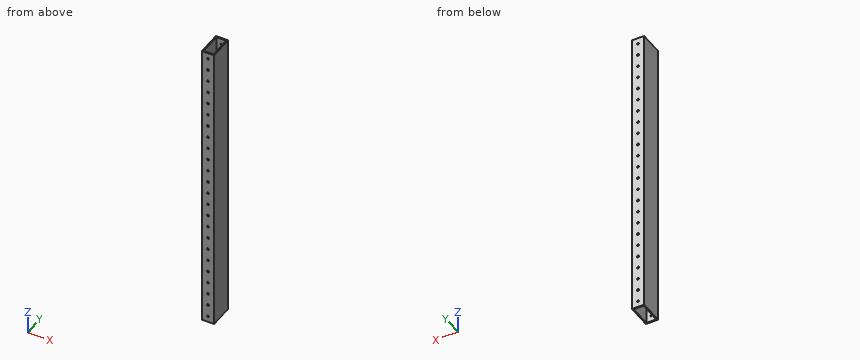
Autodesk Inventor part; units mm, degrees
ref_plane "YZ Plane" through (0, 0, 0) normal (1, 0, 0) x (0, 1, 0)
ref_plane "XZ Plane" through (0, 0, 0) normal (0, 1, 0) x (-1, 0, 0)
ref_plane "XY Plane" through (0, 0, 0) normal (0, 0, 1) x (1, 0, 0)
sketch "Sketch1" plane through (0, 0, 0) normal (0, 0, 1) x (1, 0, 0)
  line L0 (0, 0) -> (25.4, 0)
  line L1 (25.4, 0) -> (25.4, 50.8)
  line L2 (25.4, 50.8) -> (0, 50.8)
  line L3 (0, 50.8) -> (0, 0)
  line L4 (2.54, 2.54) -> (22.86, 2.54)
  line L5 (22.86, 2.54) -> (22.86, 48.26)
  line L6 (22.86, 48.26) -> (2.54, 48.26)
  line L7 (2.54, 48.26) -> (2.54, 2.54)
  dimension "d0" = 25.4
  dimension "d1" = 50.8
  dimension "d2" = 2.54
extrude "Extrusion1" add sketch "Sketch1" along normal blind 609.6
sketch "Sketch2" plane through (0, 50.8, 0) normal (0, 1, 0) x (1, 0, 0)
  line L0 (25.4, -609.6) -> (0, -609.6)
  line L1 (0, 0) -> (0, -609.6)
  point P0 (12.7, -596.9)
  point P1 (12.7, -571.5)
  point P2 (12.7, -546.1)
  point P3 (12.7, -520.7)
  point P4 (12.7, -495.3)
  point P5 (12.7, -469.9)
  point P6 (12.7, -444.5)
  point P7 (12.7, -419.1)
  point P8 (12.7, -393.7)
  point P9 (12.7, -368.3)
  point P10 (12.7, -342.9)
  point P11 (12.7, -317.5)
  point P12 (12.7, -292.1)
  point P13 (12.7, -266.7)
  point P14 (12.7, -241.3)
  point P15 (12.7, -215.9)
  point P16 (12.7, -190.5)
  point P17 (12.7, -165.1)
  point P18 (12.7, -139.7)
  point P19 (12.7, -114.3)
  point P20 (12.7, -88.9)
  point P21 (12.7, -63.5)
  point P22 (12.7, -38.1)
  point P23 (12.7, -12.7)
  dimension "d5" = 12.7
  dimension "d6" = 12.7
  dimension "d9" = 25.4
hole "Hole1" at (12.7, 50.8, 596.9) at (12.7, 50.8, 571.5) at (12.7, 50.8, 546.1) at (12.7, 50.8, 520.7) at (12.7, 50.8, 495.3) at (12.7, 50.8, 469.9) at (12.7, 50.8, 444.5) at (12.7, 50.8, 419.1) at (12.7, 50.8, 393.7) at (12.7, 50.8, 368.3) at (12.7, 50.8, 342.9) at (12.7, 50.8, 317.5) at (12.7, 50.8, 292.1) at (12.7, 50.8, 266.7) at (12.7, 50.8, 241.3) at (12.7, 50.8, 215.9) at (12.7, 50.8, 190.5) at (12.7, 50.8, 165.1) at (12.7, 50.8, 139.7) at (12.7, 50.8, 114.3) at (12.7, 50.8, 88.9) at (12.7, 50.8, 63.5) at (12.7, 50.8, 38.1) at (12.7, 50.8, 12.7) direction (0, -1, 0) diameter 4.1402 end through all
properties part number "24in2x1Extrusion" material "Aluminum 6061"
The listing builds one solid part. Answer for the finished solid, in the listing's coordinates (mm). Give positions to 0.01 mm unless a question says otherwise; leave off trailing zeros. Order: outer loops, then holes, each group sorted by start corner. A loop starts at its lowest first (then second) coordinate and runs counter-clockwise, first axis right, second up. Notation, with made-up numbers: (-23.75, -5.5) - (3.25, -5.5) arc R6 ccw to (3.25, 1.5) - close; hole circle Ø2 at (-37, 59.5). An arc over 180 degrees is marked (long way). One line per item, written item: value. Start each with the question number.
1) Given pin 1 Ø2.5 at (x, z) = (12.7, 596.9) entering from +Y, flat-ended and moving along its own axis, determine where the tip first touches the part or whether it passes through.
2) Find the intervals of material crossed by L1, parallel to X at y = 22, z = 71.5; L2, parallel to Y at x = 20, z = 339; L3, parallel to X at y = 49, z = 190, in increasing order.
3) A cutting plane is placed at B-B on y = 42.5. Give the vertices of the cut face in (x, z), then the cut area to 3 significant figures.
4) A cutting plane is placed at A-A on z = 558. Give the vertices of the cut face in (x, y).
Answer sheet:
1. pin 1: passes through
2. L1: x = 0 to 2.54, 22.86 to 25.4
2. L2: y = 0 to 2.54, 48.26 to 50.8
2. L3: x = 0 to 10.69, 14.71 to 25.4
3. outline: (0, 0) - (2.54, 0) - (2.54, 609.6) - (0, 609.6) - close; (22.86, 0) - (25.4, 0) - (25.4, 609.6) - (22.86, 609.6) - close
3. area: 3,100 mm2
4. outline: (0, 0) - (25.4, 0) - (25.4, 50.8) - (0, 50.8) - close; hole (2.54, 2.54) - (22.86, 2.54) - (22.86, 48.26) - (2.54, 48.26) - close
